```python
from build123d import *

# Parameters (mm, degrees)
BOSS_EXTRUDE1_DEPTH                                  = 5
CSK_FOR_M3_HEX_SOCKET_COUNTERSUNK_HEAD_S_D           = 3.4
CSK_FOR_M3_HEX_SOCKET_COUNTERSUNK_HEAD_S_CSINK_D     = 6.94
CSK_FOR_M3_HEX_SOCKET_COUNTERSUNK_HEAD_S_CSINK_ANGLE = 90
SKETCH5_W                                            = 1.6
SKETCH5_H                                            = 1
CUT_EXTRUDE1_DEPTH                                   = 4


with BuildPart() as part:
    # Sketch1 → Boss-Extrude1 (new body)
    with BuildSketch(Plane(origin=(0, 0, 0), x_dir=(1, 0, 0), z_dir=(0, 1, 0))):
        with BuildLine():
            Line((-8, 4.5), (8, 4.5))
            ThreePointArc((8, 4.5), (9.414213562, 3.914213562), (10, 2.5))
            Line((10, 2.5), (10, -2.5))
            ThreePointArc((10, -2.5), (9.414213562, -3.914213562), (8, -4.5))
            Line((8, -4.5), (-8, -4.5))
            ThreePointArc((-8, -4.5), (-9.414213562, -3.914213562), (-10, -2.5))
            Line((-10, -2.5), (-10, 2.5))
            ThreePointArc((-10, 2.5), (-9.414213562, 3.914213562), (-8, 4.5))
        make_face()
    extrude(amount=BOSS_EXTRUDE1_DEPTH)

    # CSK for M3 Hex Socket Countersunk Head Screw1 (through all)
    with Locations(Plane(origin=(0, 5, 0), x_dir=(1, 0, 0), z_dir=(0, 1, 0))):
        with Locations((-6, 0), (6, 0)):
            CounterSinkHole(CSK_FOR_M3_HEX_SOCKET_COUNTERSUNK_HEAD_S_D / 2, CSK_FOR_M3_HEX_SOCKET_COUNTERSUNK_HEAD_S_CSINK_D / 2, counter_sink_angle=CSK_FOR_M3_HEX_SOCKET_COUNTERSUNK_HEAD_S_CSINK_ANGLE)

    # Sketch5 → Cut-Extrude1 (cut, symmetric)
    with BuildSketch(Plane(origin=(0, 0, 0), x_dir=(0, 0, -1), z_dir=(1, 0, 0))):
        with Locations((2.5, 0.5)):
            Rectangle(SKETCH5_W, SKETCH5_H)
        with Locations((-5, 0.5)):
            Rectangle(SKETCH5_W, SKETCH5_H)
        with Locations((-2.5, 0.5)):
            Rectangle(SKETCH5_W, SKETCH5_H)
        with Locations((0, 0.5)):
            Rectangle(SKETCH5_W, SKETCH5_H)
        with Locations((5, 0.5)):
            Rectangle(SKETCH5_W, SKETCH5_H)
    extrude(amount=CUT_EXTRUDE1_DEPTH, both=True, mode=Mode.SUBTRACT)


solid = part.part
```
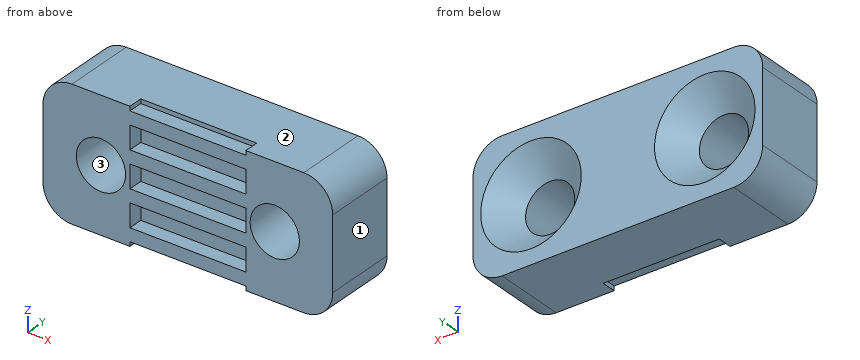
The listing builds one solid part. Answer for the finished solid, in the listing's coordinates (mm). Face numbers are marked on the shaded views. Coordinates: 2 decimals unless noted, no trailing zeros. Loops run counter-clockwise (first coordinate to the right, second up) from the corner with the lowest first, then second, coordinate; pieces in that order, holes last. Notation, with made-up numbers: (-30, -31) - (19, -31) arc R22 ccw to (19, 7) - close; hole circle Ø4 at (75.25, 86). An arc over 180 degrees is marked (long way). Use a Markdown table: item, result. Add a question column.
1) The part is cut by section B-B, the plane y = 0.7. State how many separate pieces and enclosed holes the cut face has, and give its area (3 significant figures).
2) Given pin 1 (0.8 mm diameter, centred on x = 2, y = 0.5, fed in from +Z); pin 2 (0.8 mm diameter, centred on x = 1, z = 2.5, fed in from -Y); pin 3 (0.5 mm diameter, centred on x = 0.5, y = 0.5, fed in from -Z), each flat-ended and moving along its own axis, determine where each tip first touches the part or whether it passes through.
3) The part is cut by section C-C, the plane z = 0. Give the vertices of the cut face in (x, y).
4) The mould has two halves that part along X. Classify the marked faces 1, 2 and 3: released by +X, released by -X, zero draft, split by the parting line, or undercut.
5) The part is cut by section A-A, the plane x = 6. Give the vertices of the cut face in (y, z), and give its area (3 significant figures).
6) Find the intervals of material crossed by line 1 (Z direction, x = 6, y = 1.3); line 2 (X direction, y = 0.8, z = 1.75); line 3 (Z direction, x = -4.5, y = 2), in increasing order.
7) The part is cut by section D-D, the plane y = 3.55. Give the vertices of the cut face in (x, z), and give its area (3 significant figures).
Here are the results:
| question | item | result |
|---|---|---|
| 1 | separate pieces | 1 |
| 1 | enclosed holes | 5 |
| 1 | area | 115 mm^2 |
| 2 | pin 1 | stops at z = 4.2 |
| 2 | pin 2 | stops at y = 1 |
| 2 | pin 3 | stops at z = -4.2 |
| 3 | outline | (-10, 0) - (-7.7, 0) - (-7.7, 3.23) - (-9.47, 5) - (-10, 5) - close; (-4.3, 0) - (-4, 0) - (-4, 1) - (4, 1) - (4, 0) - (4.3, 0) - (4.3, 3.23) - (2.53, 5) - (-2.53, 5) - (-4.3, 3.23) - close; (7.7, 0) - (10, 0) - (10, 5) - (9.47, 5) - (7.7, 3.23) - close |
| 4 | face 1 | released by +X |
| 4 | face 2 | zero draft |
| 4 | face 3 | undercut |
| 5 | outline | (0, -4.5) - (5, -4.5) - (5, -3.47) - (3.23, -1.7) - (0, -1.7) - close; (0, 1.7) - (3.23, 1.7) - (5, 3.47) - (5, 4.5) - (0, 4.5) - close |
| 5 | area | 24.9 mm^2 |
| 6 | line 1 | z = -4.5 to -1.7, 1.7 to 4.5 |
| 6 | line 2 | x = -10 to -4, 4 to 10 |
| 6 | line 3 | z = -4.5 to -0.8, 0.8 to 4.5 |
| 7 | outline | (-10, -2.5) arc R2 ccw to (-8, -4.5) - (8, -4.5) arc R2 ccw to (10, -2.5) - (10, 2.5) arc R2 ccw to (8, 4.5) - (-8, 4.5) arc R2 ccw to (-10, 2.5) - close; hole circle Ø4.04 at (-6, 0); hole circle Ø4.04 at (6, 0) |
| 7 | area | 151 mm^2 |
